```python
from build123d import *

# Parameters (mm, degrees)
SKETCH_1_R          = 12.5
EXTRUDE_1_DEPTH     = 4
SKETCH_2_R          = 4.5
EXTRUDE_2_DEPTH     = 2
SKETCH_3_R          = 1
CUT_EXTRUDE_3_DEPTH = 19.12456896
SKETCH_4_R          = 1
CUT_EXTRUDE_4_DEPTH = 19.668154703
SKETCH_5_R          = 4
CUT_EXTRUDE_5_DEPTH = 2
SKETCH_6_R          = 12.5
EXTRUDE_3_DEPTH     = 4
SKETCH_7_R          = 1
CUT_EXTRUDE_6_DEPTH = 4


with BuildPart() as part:
    # 草图1 → 凸台-拉伸1 (new body)
    with BuildSketch(Plane.XY):
        Circle(SKETCH_1_R)
    extrude(amount=EXTRUDE_1_DEPTH)

    # 草图2 → 凸台-拉伸2 (add)
    with BuildSketch(Plane.XY.offset(4)):
        Circle(SKETCH_2_R)
    extrude(amount=EXTRUDE_2_DEPTH)

    # 草图3 → 切除-拉伸3 (cut, through all)
    with BuildSketch(Plane.XY.offset(4)):
        with Locations((4.955921216, 5)):
            Circle(SKETCH_3_R)
        with Locations(Location((4.955921216, -5, 0), (0, 0, 180))):
            Circle(SKETCH_3_R)
        with Locations((-4.955921216, -5)):
            Circle(SKETCH_3_R)
        with Locations(Location((-4.955921216, 5, 0), (0, 0, 180))):
            Circle(SKETCH_3_R)
    extrude(amount=-CUT_EXTRUDE_3_DEPTH, mode=Mode.SUBTRACT)

    # 草图4 → 切除-拉伸4 (cut, through all)
    with BuildSketch(Plane.XY.offset(6)):
        Circle(SKETCH_4_R)
    extrude(amount=-CUT_EXTRUDE_4_DEPTH, mode=Mode.SUBTRACT)

    # 草图5 → 切除-拉伸5 (cut)
    with BuildSketch(Plane.XY.offset(6)):
        Circle(SKETCH_5_R)
    extrude(amount=-CUT_EXTRUDE_5_DEPTH, mode=Mode.SUBTRACT)

    # 草图6 → 凸台-拉伸3 (add)
    with BuildSketch(Plane(origin=(0, 0, 0), x_dir=(-1, 0, 0), z_dir=(0, 0, -1))):
        with Locations(Location((0, 0, 0), (0, 0, 180))):
            Circle(SKETCH_6_R)
    extrude(amount=-EXTRUDE_3_DEPTH)

    # 草图7 → 切除-拉伸6 (cut)
    with BuildSketch(Plane(origin=(0, 0, 0), x_dir=(-1, 0, 0), z_dir=(0, 0, -1))):
        with Locations((7.071067812, 0)):
            Circle(SKETCH_7_R)
        Circle(SKETCH_7_R)
        with Locations((0, 7.071067812)):
            Circle(SKETCH_7_R)
        with Locations((-7.071067812, 0)):
            Circle(SKETCH_7_R)
        with Locations((0, -7.071067812)):
            Circle(SKETCH_7_R)
    extrude(amount=-CUT_EXTRUDE_6_DEPTH, mode=Mode.SUBTRACT)


solid = part.part
```
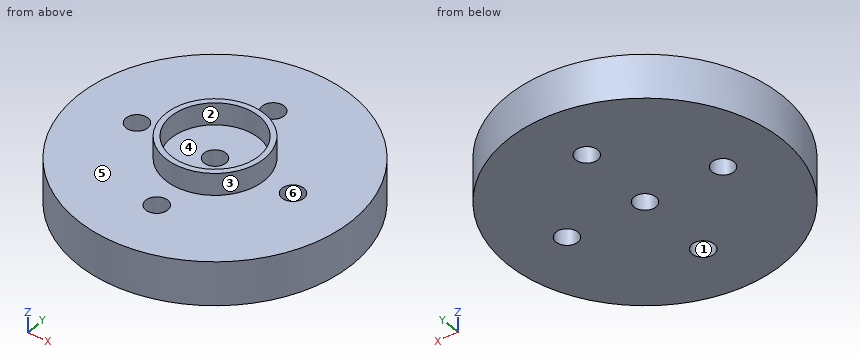
Can you work these out from the model? Positions are in its coordinate system, mm. Face numbers are marked on the shaded views. A direction names the side the tool comes from. Round coordinates to 2 decimals unless told otherwise and drop trailing zeros. Loops run counter-clockwise (first coordinate to the right, second up) from the corner with the lowest first, then second, coordinate; pieces in that order, holes last. Notation, with made-up numbers: (0, 33.25) -> (55, 33.25) arc R17 cw to (55, 49.25) -> close; hole circle Ø4 at (-18, -5.75). An arc over 180 degrees is marked (long way). One line per item, written item: value. Start each with the question number.
1. If we section it at A-A, the plane x = 0: Write out the boundary of the cut face in (y, z), then the cut area to 3 significant figures.
2. For pin 1 (2.5 mm diameter, centred on x = 7.07, y = 0, fed in from -Z); pin 2 (1 mm diameter, centred on x = 4, y = 4, fed in from +Z); pin 3 (1.2 mm diameter, centred on x = -7.07, y = 0, fed in from +Z), each with a flat end and sliding along its axis, tell me the tip position at first contact or that it passes through.
3. If we section it at C-C, the plane x = 7.5: Write out the boundary of the cut face in (y, z).
4. If I drill on probe 1 along Y at (x, z) = (0, 2.85); probe 2 along X at (y, z) = (0.75, 1.25); probe 3 along Y at (x, z) = (0.25, 1.6), over which ranges is the centre line in solid material (lowest first)?
5. If we mould it in two halves opening along Y, with no side actions, what happens to the marked faces 3, 4, 5 and 6? For each: pulls with the +Y half, pulls with the -Y half, needs draft (parallel to the pull), parting line crosses it, or undercut.
6. If we section it at D-D, the plane z = 5.65: Write out the boundary of the cut face in (x, y), then the cut area to 3 significant figures.
7. For the marked faces 1 and 2, which set-ups out of +Z, -Z, +X, -X, +Y, -Y let a thin tool reach every point of the face, with its end or its side?
Calculated:
1. outline: (-12.5, 0) -> (-8.07, 0) -> (-8.07, 4) -> (-12.5, 4) -> close; (-6.07, 0) -> (-1, 0) -> (-1, 4) -> (-4, 4) -> (-4, 6) -> (-4.5, 6) -> (-4.5, 4) -> (-6.07, 4) -> close; (1, 0) -> (6.07, 0) -> (6.07, 4) -> (4.5, 4) -> (4.5, 6) -> (4, 6) -> (4, 4) -> (1, 4) -> close; (8.07, 0) -> (12.5, 0) -> (12.5, 4) -> (8.07, 4) -> close
1. area: 78.0 mm²
2. pin 1: stops at z = 0
2. pin 2: stops at z = 4
2. pin 3: passes through
3. outline: (-10, 0) -> (-0.9, 0) -> (-0.9, 4) -> (-10, 4) -> close; (0.9, 0) -> (10, 0) -> (10, 4) -> (0.9, 4) -> close
4. probe 1: y = -12.5 to -8.07, -6.07 to -1, 1 to 6.07, 8.07 to 12.5
4. probe 2: x = -12.48 to -7.73, -6.41 to -0.66, 0.66 to 6.41, 7.73 to 12.48
4. probe 3: y = -12.5 to -8.04, -6.1 to -0.97, 0.97 to 6.1, 8.04 to 12.5
5. face 3: parting line crosses it
5. face 4: undercut
5. face 5: needs draft
5. face 6: undercut
6. outline: circle Ø9 at (0, 0); hole circle Ø8 at (0, 0)
6. area: 13.4 mm²
7. face 1: +Z, -Z
7. face 2: +Z
